from build123d import *

# Parameters (mm, degrees)
SKETCH1_W                       = 32.004
SKETCH1_H                       = 98.1456
SKETCH2_R                       = 31.877
BOSS_EXTRUDE1_DEPTH             = 8.2296
SKETCH3_R                       = 15.0368
BOSS_EXTRUDE2_DEPTH             = 4.7625
SKETCH4_R                       = 31.877
BOSS_EXTRUDE3_DEPTH             = 8.2296
SKETCH5_R                       = 9.525
BOSS_EXTRUDE4_DEPTH             = 4.064
SKETCH6_R                       = 4
BOSS_EXTRUDE5_DEPTH             = 31.5
CUT_EXTRUDE1_REACH              = 31.204
F_21_0_159_DIAMETER_HOLE1_D     = 4.0386
F_21_0_159_DIAMETER_HOLE1_DEPTH = 13.6144
F_21_0_159_DIAMETER_HOLE1_TIP   = 1.213317848
CHAMFER1_SIZE2                  = 1.016
CHAMFER1_SIZE                   = 1.015999998
FILLET1_R                       = 0.254
FILLET2_R                       = 1


with BuildPart() as part:
    # Sketch1 → Revolve1 (revolve)
    with BuildSketch(Plane.XZ.offset(-109.2962)):
        with Locations((51.562, -38.2524)):
            Rectangle(SKETCH1_W, SKETCH1_H)
    revolve(axis=Axis((35.56, 109.2962, 10.8204), (0, 0, -1)))

    # Sketch2 → Boss-Extrude1 (add)
    with BuildSketch(Plane(origin=(0, 0, -87.3252), x_dir=(-1, 0, 0), z_dir=(0, 0, -1))):
        with Locations((-35.56, 109.2962)):
            Circle(SKETCH2_R)
    extrude(amount=BOSS_EXTRUDE1_DEPTH)

    # Sketch3 → Boss-Extrude2 (add)
    with BuildSketch(Plane(origin=(0, 0, -95.5548), x_dir=(-1, 0, 0), z_dir=(0, 0, -1))):
        with Locations((-35.56, 109.2962)):
            Circle(SKETCH3_R)
    extrude(amount=BOSS_EXTRUDE2_DEPTH)

    # Sketch4 → Boss-Extrude3 (add)
    with BuildSketch(Plane.XY.offset(10.8204)):
        with Locations((35.56, 109.2962)):
            Circle(SKETCH4_R)
    extrude(amount=BOSS_EXTRUDE3_DEPTH)

    # Sketch5 → Boss-Extrude4 (add)
    with BuildSketch(Plane.XY.offset(19.05)):
        with Locations((35.56, 109.2962)):
            Circle(SKETCH5_R)
    extrude(amount=BOSS_EXTRUDE4_DEPTH)

    # Sketch6 → Boss-Extrude5 (add)
    with BuildSketch(Plane.XY.offset(23.114)):
        with Locations((35.56, 109.2962)):
            Circle(SKETCH6_R)
    extrude(amount=BOSS_EXTRUDE5_DEPTH)

    # Sketch7 → Cut-Extrude1 (cut, up to next)
    with BuildSketch(Plane(origin=(38.36, 0, 0), x_dir=(0, -1, 0), z_dir=(-1, 0, 0)), mode=Mode.PRIVATE) as cut_extrude1_sk1:
        with BuildLine():
            Line((-108.2462, 27.1), (-108.2462, 45.1))
            ThreePointArc((-108.2462, 45.1), (-109.2962, 46.15), (-110.3462, 45.1))
            Line((-110.3462, 45.1), (-110.3462, 27.1))
            ThreePointArc((-110.3462, 27.1), (-109.2962, 26.05), (-108.2462, 27.1))
        make_face()
    cut_extrude1_tool1 = extrude(cut_extrude1_sk1.sketch, amount=-CUT_EXTRUDE1_REACH, mode=Mode.PRIVATE) & part.part
    add(cut_extrude1_tool1.solids().sort_by_distance((38.36, 109.2962, 36.1))[0], mode=Mode.SUBTRACT)

    # Sketch8 → Revolve2 (revolve)
    with BuildSketch(Plane.XZ.offset(-120.503559639)):
        Polygon((58.485090683, -95.5548), (54.167090681, -95.5548), (54.167090681, -97.802699998), (56.285090681, -97.802699998), (58.485090683, -95.602699996), align=None)
    revolve(axis=Axis((54.167090681, 120.503559639, -95.5548), (0, 0, -1)))

    # Sketch9 → Revolve3 (revolve)
    with BuildSketch(Plane.XZ.offset(-127.903290683)):
        Polygon((51.085359639, -95.5548), (46.767359637, -95.5548), (46.767359637, -97.802699998), (48.885359637, -97.802699998), (51.085359639, -95.602699996), align=None)
    revolve(axis=Axis((46.767359637, 127.903290683, -95.5548), (0, 0, -1)))

    # #21 (0.159) Diameter Hole1
    with Locations(Plane.XY.offset(19.05)):
        with Locations((10.16, 109.2962), (60.96, 109.2962)):
            Hole(F_21_0_159_DIAMETER_HOLE1_D / 2, depth=F_21_0_159_DIAMETER_HOLE1_DEPTH)
            with Locations((0, 0, -(F_21_0_159_DIAMETER_HOLE1_DEPTH + F_21_0_159_DIAMETER_HOLE1_TIP / 2))):  # 118° drill point
                Cone(0, F_21_0_159_DIAMETER_HOLE1_D / 2, F_21_0_159_DIAMETER_HOLE1_TIP, mode=Mode.SUBTRACT)

    # Chamfer1
    chamfer1_edges = [part.edges().sort_by_distance(p)[0] for p in [
        (26.035, 109.2962, 23.114),
    ]]
    chamfer(chamfer1_edges, length=CHAMFER1_SIZE, length2=CHAMFER1_SIZE2)

    # Fillet1
    fillet1_edges = [part.edges().sort_by_distance(p)[0] for p in [
        (31.56, 109.2962, 54.614),
    ]]
    fillet(fillet1_edges, radius=FILLET1_R)

    # Fillet2
    fillet2_edges = [part.edges().sort_by_distance(p)[0] for p in [
        (50.5968, 109.2962, -100.3173),
        (3.683, 109.2962, 19.05),
        (67.437, 109.2962, -95.5548),
    ]]
    fillet(fillet2_edges, radius=FILLET2_R)


solid = part.part
The listing builds one solid part. Answer for the finished solid, in the listing's coordinates (mm). A direction names the side the tool comes from. Coordinates: 2 decimals unless noted, no trailing zeros. Order: outer loops, then holes, each group sorted by start corner. A loop starts at its lowest first (then second) coordinate and runs counter-clockwise, first axis right, second up.
Q1. Consider line 1 (Z direction, x = 33.5, y = 116); line 2 (Z direction, x = 34, y = 89.5); line 3 (Y direction, x = 10, z = 9). Determine where each line is inside the solid, lowest interval first.
Q2. A cutting plane is placed at D-D, the plane z = -33. Write down the section's boundary in (x, y).
Q3. For a pull along Y with two mould halves and no side action, classify faces 4 (the face through (6.114, 97.087, -90.889)), 5 (the face through (54, 120, -97.803)), 6 (the face through (10.084, 108.954, 4.433)) as pulls with the +Y half, pulls with the -Y half, needs draft (parallel to the pull), parting line crosses it, or undercut.
Q4. A cutting plane is placed at C-C, the plane z = 39. Write down the section's boundary in (x, y), and give its area (3 significant figures).
Q5. Given P1, Ø6, axis at y = 120.5, z = -63, coming from the -X side; P2, Ø12, axis at y = 100, z = -22, coming from the +X side; P3, Ø5, axis at x = 50, z = -37, coming from the +Y side, each flat-ended and moving along its own axis, determine where each tip first touches the part or whether it passes through.
Q6. A cutting plane is placed at B-B, the plane z = 13. Write down the section's boundary in (x, y).
Q7. Which of the six approach directions +Z, -Z, +X, -X, +Y, -Y give full straight-line access (tool end or side, diameter ignored) to faces 1 (the face through (34.69, 105.39, 38.52)), 2 (the face through (38.82, 94.617, -97.41)), 3 (the face through (47, 128, -97.803))?
Answers follow:
1. line 1: z = -100.32 to 23.11
1. line 2: z = -95.55 to 19.05
1. line 3: y = 90.04 to 107.28, 111.31 to 128.56
2. outline: circle Ø64.01 at (35.56, 109.3)
3. face 4: parting line crosses it
3. face 5: needs draft
3. face 6: undercut
4. outline: (38.36, 108.25) - (38.36, 110.35) - (39.42, 110.35) arc R4 ccw (long way) to (39.42, 108.25) - close
4. area: 47.8 mm2
5. P1: stops at x = 4.63
5. P2: stops at x = 67.39
5. P3: stops at y = 138.99
6. outline: circle Ø63.75 at (35.56, 109.3); hole circle Ø4.04 at (10.16, 109.3); hole circle Ø4.04 at (60.96, 109.3)
7. face 1: +Z
7. face 2: -Z
7. face 3: -Z, +X, -X, +Y
